Source: CAD feature listing. Evaluate the final solid. Frame: model axes, mm. A direction names the side the tool comes from. Give positions to 0.01 mm unless a question says otherwise; leave off trailing zeros. Write each loop counter-clockwise with the first axis right and the second up, starting at its lowest first coordinate (ties: lowest second). Pieces come first, ordered by that corner, then holes.
```python
from build123d import *

# Parameters (mm, degrees)
SKETCH_1_R             = 15.1
EXTRUDE_1_DEPTH        = 2.15
SKETCH_2_R             = 12.49
EXTRUDE_2_DEPTH        = 5
SKETCH_3_R             = 7.265
EXTRUDE_3_DEPTH        = 3.7
SKETCH_4_R             = 16.95
EXTRUDE_4_DEPTH        = 1
SKETCH_5_R             = 1.25
CUT_EXTRUDE_1_DEPTH    = 1
FILLET_1_R             = 0.3
CHAMFER_1_SIZE         = 0.3
HOLE_WIZARD_M2_1_D     = 1.6
HOLE_WIZARD_M2_1_DEPTH = 5.2
HOLE_WIZARD_M2_1_TIP   = 0.480688495


with BuildPart() as part:
    # 草图1 → 凸台-拉伸1 (new body)
    with BuildSketch(Plane(origin=(0, 0, 0), x_dir=(1, 0, 0), z_dir=(0, 1, 0))):
        Circle(SKETCH_1_R)
    extrude(amount=EXTRUDE_1_DEPTH)

    # 草图2 → 凸台-拉伸2 (add)
    with BuildSketch(Plane(origin=(0, 2.15, 0), x_dir=(1, 0, 0), z_dir=(0, 1, 0))):
        Circle(SKETCH_2_R)
    extrude(amount=EXTRUDE_2_DEPTH)

    # 草图3 → 凸台-拉伸3 (add)
    with BuildSketch(Plane(origin=(0, 7.15, 0), x_dir=(1, 0, 0), z_dir=(0, 1, 0))):
        Circle(SKETCH_3_R)
    extrude(amount=EXTRUDE_3_DEPTH)

    # 草图4 → 凸台-拉伸4 (add)
    with BuildSketch(Plane(origin=(0, 0, 0), x_dir=(-1, 0, 0), z_dir=(0, -1, 0))):
        Circle(SKETCH_4_R)
    extrude(amount=EXTRUDE_4_DEPTH)

    # 草图5 → 切除-拉伸1 (cut)
    with BuildSketch(Plane(origin=(0, 10.85, 0), x_dir=(1, 0, 0), z_dir=(0, 1, 0))):
        Circle(SKETCH_5_R)
    extrude(amount=-CUT_EXTRUDE_1_DEPTH, mode=Mode.SUBTRACT)

    # 圆角1
    fillet_1_edges = [part.edges().sort_by_distance(p)[0] for p in [
        (-7.265, 10.85, 0),
    ]]
    fillet(fillet_1_edges, radius=FILLET_1_R)

    # 倒角1
    chamfer_1_edges = [part.edges().sort_by_distance(p)[0] for p in [
        (16.95, 0, 0),
        (-15.1, 2.15, 0),
        (-12.49, 7.15, 0),
    ]]
    chamfer(chamfer_1_edges, length=CHAMFER_1_SIZE)

    # M2 螺纹孔1
    with Locations(Plane(origin=(0, 7.15, 0), x_dir=(1, 0, 0), z_dir=(0, 1, 0))):
        with Locations((5.25, 9.09326674), (10.5, 0), (5.25, -9.09326674), (-5.25, -9.09326674), (-10.5, 0), (-5.25, 9.09326674)):
            Hole(HOLE_WIZARD_M2_1_D / 2, depth=HOLE_WIZARD_M2_1_DEPTH)
            with Locations((0, 0, -(HOLE_WIZARD_M2_1_DEPTH + HOLE_WIZARD_M2_1_TIP / 2))):  # 118° drill point
                Cone(0, HOLE_WIZARD_M2_1_D / 2, HOLE_WIZARD_M2_1_TIP, mode=Mode.SUBTRACT)


solid = part.part
```
1. Section query B-B (y = 9). Return loops of the section in (x, z) (3 decimals).
2. Line query: probe 1 along Z at (x, y) = (5.25, 4.9); probe 2 along Y at (x, z) = (-9.5, 6); probe 3 along Z at (x, y) = (0, 10.1) (3 decimals). Output: solid intervals per line, ascending.
3. Section query C-C (y = 0.5). Return loops of the section in (x, z), plus the area to 3 significant figures.
4. Pin query (flat end, axial travel): P1, Ø1.3, axis at x = 5.25, z = -9.09, coming from the +Y side; P2, Ø2, axis at x = 0, z = 0, coming from the +Y side; P3, Ø1.8, axis at x = 10.5, z = 0, coming from the +Y side. Return the tip coordinate at first contact, or that it passes through.
5. Section query A-A (y = 5.75). Return loops of the section in (x, z), plus the area to 3 significant figures.
6. Access query for faces 1 (the flat face through (-0.1, 10.85, 1.5)), 2 (the flat face through (5.25, 7.15, 5.25)). Directions: +Z, -Z, +X, -X, +Y, -Y. A direction counts if a zero-diameter tool reaches every point of the face in a straight line with its end or side. Return the directions, or none.
7. Pull-direction query (Z, two-part tool) for faces 3 (the flat face through (-10, 2.15, 8)), 4 (the cylindrical face through (-5.765, 8.826, 4.421)), 5 (the conical face through (5.22, 1.553, 9.229)), 6 (the cylindrical face through (6.05, 4.51, -9.13)); classes: pulls with the +Z half, pulls with the -Z half, needs draft (parallel to the pull), parting line crosses it, or undercut.
The answers:
1. outline: circle Ø14.53 at (0, 0)
2. probe 1: z = -11.33 to -9.89, -8.29 to 8.29, 9.89 to 11.33
2. probe 2: y = -1 to 7.15
2. probe 3: z = -7.265 to -1.25, 1.25 to 7.265
3. outline: circle Ø30.2 at (0, 0)
3. area: 716 mm2
4. P1: stops at y = 1.86
4. P2: stops at y = 9.85
4. P3: stops at y = 7.15
5. outline: circle Ø24.98 at (0, 0); hole circle Ø1.6 at (-10.5, 0); hole circle Ø1.6 at (-5.25, -9.09); hole circle Ø1.6 at (-5.25, 9.09); hole circle Ø1.6 at (5.25, -9.09); hole circle Ø1.6 at (5.25, 9.09); hole circle Ø1.6 at (10.5, 0)
5. area: 478 mm2
6. face 1: +Z, -Z, +X, -X, +Y
6. face 2: +Y
7. face 3: needs draft
7. face 4: parting line crosses it
7. face 5: undercut
7. face 6: undercut
